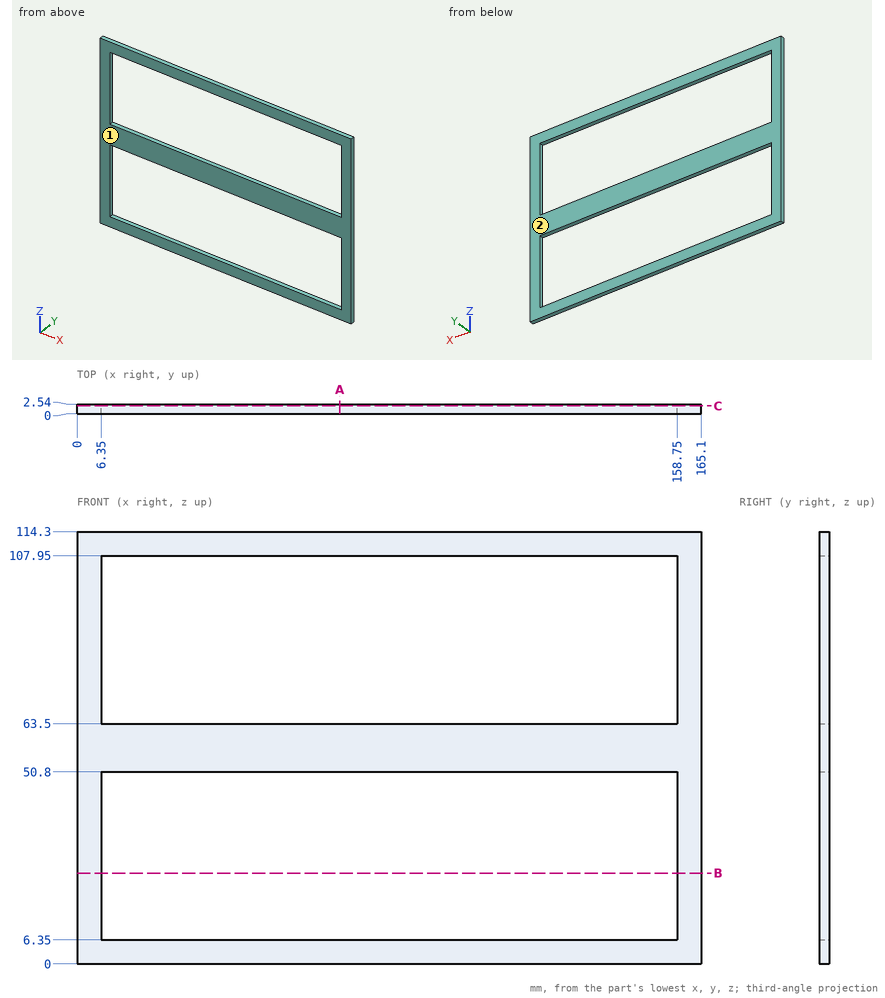
Geometry check sheet. Reference: drawing and pictorial views, mm from the part's lowest x, y, z. Give positions to 0.01 mm unless a question says otherwise; leave off trailing zeros. Write each loop counter-clockwise with the first axis right and the second up, starting at its lowest first coordinate (ties: lowest second). Pieces come first, ordered by that corner, then holes.
Item 1: Cross-section at C-C (y = 2.05). Enter the section's corners in (x, z), and give its area (3 significant figures).
Item 2: Cross-section at A-A (x = 69.5). Enter the section's corners in (y, z).
Item 3: Cross-section at B-B (z = 24). Enter the section's corners in (x, y).
Item 4: Scan lines: L1, parallel to Z at x = 89, y = 1.2; L2, parallel to X at y = 1.9, z = 18.5. Record each from-to range of solid material in increasing order.
Item 5: Draft check along Y on the marked faces 1 and 2. Enter one of: released by +Y, released by -Y, zero draft, split by the parting line, or undercut.
Report:
1. outline: (0, 0) - (165.1, 0) - (165.1, 114.3) - (0, 114.3) - close; hole (6.35, 6.35) - (158.75, 6.35) - (158.75, 50.8) - (6.35, 50.8) - close; hole (6.35, 63.5) - (158.75, 63.5) - (158.75, 107.95) - (6.35, 107.95) - close
1. area: 5,320 mm2
2. outline: (0, 0) - (2.54, 0) - (2.54, 6.35) - (0, 6.35) - close; (0, 50.8) - (2.54, 50.8) - (2.54, 63.5) - (0, 63.5) - close; (0, 107.95) - (2.54, 107.95) - (2.54, 114.3) - (0, 114.3) - close
3. outline: (0, 0) - (6.35, 0) - (6.35, 2.54) - (0, 2.54) - close; (158.75, 0) - (165.1, 0) - (165.1, 2.54) - (158.75, 2.54) - close
4. L1: z = 0 to 6.35, 50.8 to 63.5, 107.95 to 114.3
4. L2: x = 0 to 6.35, 158.75 to 165.1
5. face 1: released by -Y
5. face 2: released by +Y
